CAD build for the part. Positions are in the model's coordinates, mm. A direction names the side the tool comes from. Coordinates: 2 decimals unless noted, no trailing zeros. Write each loop counter-clockwise with the first axis right and the second up, starting at its lowest first coordinate (ties: lowest second). Pieces come first, ordered by that corner, then holes. Notation, with made-up numbers: (-1, 11) - (47, 11) arc R21 cw to (47, 24) - close; hole circle Ø7 at (9, 19). An arc over 180 degrees is marked (long way). Answer in a Markdown table with one row per item. Add a question column.
Q1. Two-plate mould, pull along X, no slides. Class faces 3 (the cylindrical face through (-4.336, 2.028, 19.524)), 4 (the cylindrical face through (-3, 29, 11)), 5 (the flat face through (13, 4, -5)): +X half, -X half, draft (parallel to the pull), parting line (faces both ways), or undercut.
Q2. Pin check, flat tips, straight feed: pin 1 (5 mm diameter, centred on x = 7.5, z = 14, fed in from +Y); pin 2 (9 mm diameter, centred on x = -3, z = 2, fed in from +Y); pin 3 (5 mm diameter, centred on x = -3, y = 43.5, fed in from -Z); pin 4 (10 mm diameter, centred on y = 17, z = -0.5, fed in from +X). Stop position of each tip, or through.
Q3. Band-saw the part on D-D (x = 9.5). List the corners of the cut face in (y, z).
Q4. Band-saw the part on B-B (y = 29). List the corners of the cut face in (x, z).
Q5. Band-saw the part on C-C (z = -7). List the corners of the cut face in (x, y) (3 decimals).
Q6. Band-saw the part on A-A (x = 0). List the corners of the cut face in (y, z), and give its area (3 significant figures).
Q7. 3-axis set-ups, long thin cutter, end or side, ignore diameter. For faces 1 (the flat face through (0, 6, 0)), 2 (the flat face through (0, 50, 9)): which of +Z, -Z, +X, -X, +Y, -Y reach the whole face in a straight line?
Q8. Drill centre lines: line 1 along Z through (x, y) = (0, 40.5); line 2 along Y through (x, z) = (0, 10); line 3 along Y through (x, z) = (3.5, -17.5). Where is each one in solid material? Low to high. Write a range as from..to.
```python
from build123d import *

# Parameters (mm, degrees)
SKETCH001_R = 3
HOLE_DEPTH  = 170.997689


with BuildPart() as part:
    # Sketch → Revolution (revolve)
    with BuildSketch(Plane.XY):
        Polygon((0, 0), (20, 0), (20, 4), (13.75, 4), (13.75, 50), (8.75, 50), (8.75, 6), (0, 6), align=None)
    revolve(axis=Axis((0, 0, 0), (0, 1, 0)))

    # Sketch001 → Hole (cut, through all)
    with BuildSketch(Plane.XY):
        with Locations((0, 29)):
            Circle(SKETCH001_R)
    hole = extrude(amount=-HOLE_DEPTH, mode=Mode.SUBTRACT)

    # Mirrored: Hole across XY
    add(hole.mirror(Plane.XY), mode=Mode.SUBTRACT)


solid = part.part
```
Checked values:
| question | item | result |
|---|---|---|
| 1 | face 3 | parting line |
| 1 | face 4 | undercut |
| 1 | face 5 | draft |
| 2 | pin 1 | stops at y = 50 |
| 2 | pin 2 | stops at y = 6 |
| 2 | pin 3 | stops at z = -13.74 |
| 2 | pin 4 | stops at x = 13.75 |
| 3 | outline | (0, -17.6) - (4, -17.6) - (4, -9.94) - (50, -9.94) - (50, 9.94) - (4, 9.94) - (4, 17.6) - (0, 17.6) - close |
| 4 | outline | (-3, -13.42) - (-3, -8.22) arc R8.75 cw to (-3, 8.22) - (-3, 13.42) arc R13.75 ccw to start; (3, -13.42) arc R13.75 ccw to (3, 13.42) - (3, 8.22) arc R8.75 cw to (3, -8.22) - close |
| 5 | outline | (-18.735, 0) - (18.735, 0) - (18.735, 4) - (11.835, 4) - (11.835, 50) - (5.25, 50) - (5.25, 6) - (-5.25, 6) - (-5.25, 50) - (-11.835, 50) - (-11.835, 4) - (-18.735, 4) - close |
| 6 | outline | (0, -20) - (4, -20) - (4, -13.75) - (26, -13.75) - (26, -8.75) - (6, -8.75) - (6, 8.75) - (26, 8.75) - (26, 13.75) - (4, 13.75) - (4, 20) - (0, 20) - close; (32, -13.75) - (50, -13.75) - (50, -8.75) - (32, -8.75) - close; (32, 8.75) - (50, 8.75) - (50, 13.75) - (32, 13.75) - close |
| 6 | area | 595 mm² |
| 7 | face 1 | +Y |
| 7 | face 2 | +Z, -Z, +X, -X, +Y |
| 8 | line 1 | z = -13.75..-8.75, 8.75..13.75 |
| 8 | line 2 | y = 0..26, 32..50 |
| 8 | line 3 | y = 0..4 |
